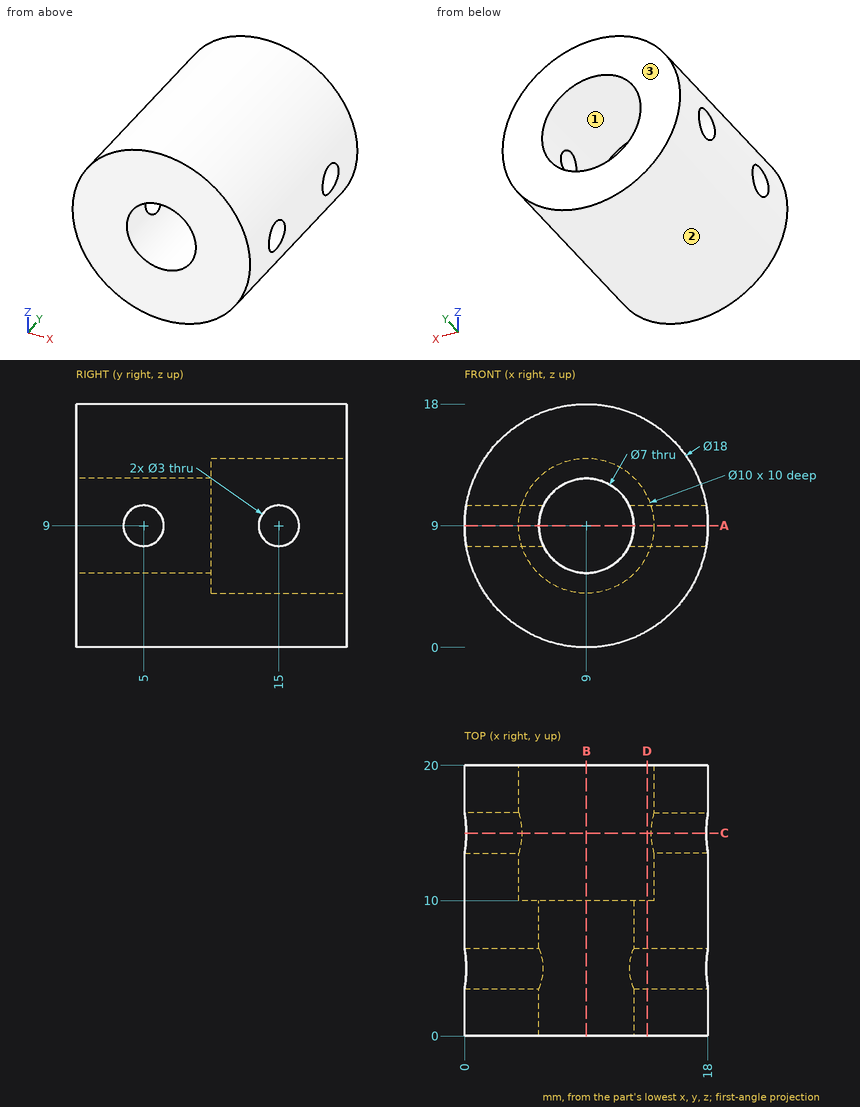
For this review, use the dimensioned drawing (mm, ordinates from the lowest corner) and the shaded views. Round coordinates to 2 decimals unless told otherwise and drop trailing zeros. Order: outer loops, then holes, each group sorted by start corner. A loop starts at its lowest first (then second) coordinate and runs counter-clockwise, first axis right, second up. Notation, with made-up numbers: (16, 12) -> (44, 12) arc R23 cw to (44, 37) -> close; hole circle Ø1 at (61.25, 57.5). An arc over 180 degrees is marked (long way). One line per item, written item: value. Start each with the question number.
Q1. Take a section at C-C (y = 15). Write out the cut boundary in (x, z).
Q2. Wall thickness on line 1 (Y direction, x = 12, z = 11.75); line 2 (Y direction, x = 17, z = 8); line 3 (X direction, y = 2.25, z = 11.25): over which ranges is each line inside the solid? List them lowest first.
Q3. Mouldability with a two-part tool opening along Z and no side actions: class the marked faces 1, 2 and 3 as released by +Z, released by -Z, zero draft, split by the parting line, or undercut.
Q4. Take a section at B-B (x = 9). Write out the cut boundary in (y, z), and give its area (3 significant figures).
Q5. Clearance check with flat-ended pins moving along their axes: pin 1 Ø2 at (x, y) = (13.5, 14.5) entering from -Z; pin 2 Ø1 at (x, y) = (10.5, 7.5) entering from +Z; pin 3 Ø2.5 at (y, z) = (5, 9) entering from +X; pin 4 Ø2 at (x, y) = (4.5, 7) entering from +Z. State where each tip first meets the part, or that it passes through.
Q6. Take a section at D-D (x = 13.5). Write out the cut boundary in (y, z).
Q7. Take a section at A-A (z = 9). Write out the cut boundary in (x, y), and give its area (3 significant figures).
Reported:
1. outline: (0.13, 7.5) arc R9 ccw to (17.87, 7.5) -> (13.77, 7.5) arc R5 cw to (4.23, 7.5) -> close; (0.13, 10.5) -> (4.23, 10.5) arc R5 cw to (13.77, 10.5) -> (17.87, 10.5) arc R9 ccw to start
2. line 1: y = 0 to 10
2. line 2: y = 0 to 3.88, 6.12 to 13.88, 16.12 to 20
2. line 3: x = 0.29 to 6.32, 11.68 to 17.71
3. face 1: undercut
3. face 2: split by the parting line
3. face 3: zero draft
4. outline: (0, 0) -> (20, 0) -> (20, 4) -> (10, 4) -> (10, 5.5) -> (0, 5.5) -> close; (0, 12.5) -> (10, 12.5) -> (10, 14) -> (20, 14) -> (20, 18) -> (0, 18) -> close
4. area: 190 mm2
5. pin 1: stops at z = 0.71
5. pin 2: stops at z = 17.94
5. pin 3: passes through
5. pin 4: stops at z = 17.29
6. outline: (0, 1.21) -> (20, 1.21) -> (20, 6.82) -> (10, 6.82) -> (10, 11.18) -> (20, 11.18) -> (20, 16.79) -> (0, 16.79) -> close; hole circle Ø3 at (5, 9)
7. outline: (0, 0) -> (5.5, 0) -> (5.5, 3.5) -> (0, 3.5) -> close; (0, 6.5) -> (5.5, 6.5) -> (5.5, 10) -> (4, 10) -> (4, 13.5) -> (0, 13.5) -> close; (0, 16.5) -> (4, 16.5) -> (4, 20) -> (0, 20) -> close; (12.5, 0) -> (18, 0) -> (18, 3.5) -> (12.5, 3.5) -> close; (12.5, 6.5) -> (18, 6.5) -> (18, 13.5) -> (14, 13.5) -> (14, 10) -> (12.5, 10) -> close; (14, 16.5) -> (18, 16.5) -> (18, 20) -> (14, 20) -> close
7. area: 133 mm2
